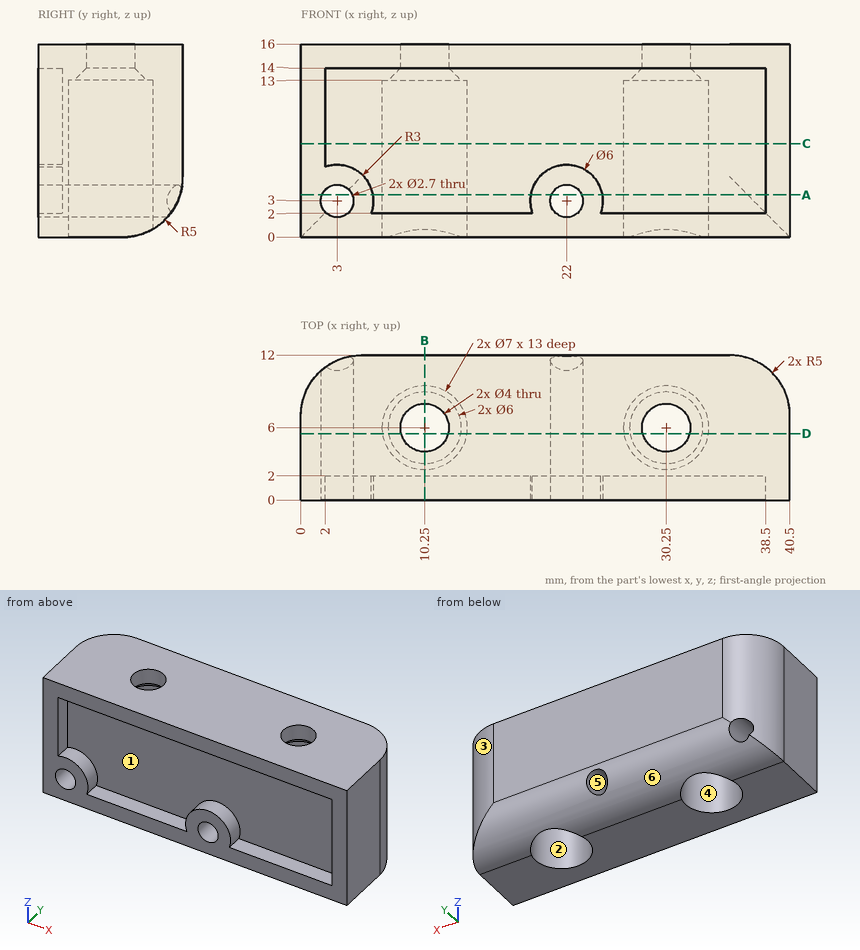
Job drawing, mm, ordinate dimensions from the low corner. One solid piece. A direction names the side the tool comes from. Round coordinates to 2 decimals unless told otherwise and drop trailing zeros. Write each loop counter-clockwise with the first axis right and the second up, starting at its lowest first coordinate (ties: lowest second). Pieces come first, ordered by that corner, then holes. Notation, with made-up numbers: M -21,-33.75 L 37,-33.75 A8 ccw 37,-27.75 Z; hole C 35.5,-12 d10. An arc over 180 degrees is marked long. Return JSON: item names as keys, results as strings. Group by question number.
(1) Two-plate mould, pull along Z, no slides. Class the marked faces 4, 5 and 6: +Z half, -Z half, draft (parallel to the pull), parting line (faces both ways), or undercut.
(2) Saw through at C-C on z = 7.75. Write the cut outline in (x, y), then the cut area to 3 significant figures.
(3) Drill centre lines: probe 1 along X at (y, z) = (1.25, 8); probe 2 along Y at (x, z) = (10.25, 8); probe 3 along X at (y, z) = (6.75, 4.5). Where is each one in solid material? Low to high.
(4) Saw through at D-D on y = 5.5. Count the separate pieces of the cut face and the enclosed holes in it, then the cut area to 3 significant figures.
(5) Saw through at A-A on z = 3.5. Write the cut outline in (x, y).
(6) Which spindle directions (+Z, -Z, +X, -X, +Y, -Y) get a long thin tool onto all of the face, cutting with end or side? Do the marked faces 1, 2 and 3. Say none if no direction does.
(7) Pin check, flat tips, straight feed: pin 1 Ø6.5 at (x, y) = (30.25, 6) entering from +Z; pin 2 Ø1 at (x, y) = (4, 9.5) entering from -Z; pin 3 Ø4.5 at (x, z) = (3, 3) entering from +Y; pin 4 Ø6 at (x, z) = (32, 7) entering from -Y. Stop position of each tip, or through.
(8) Saw through at B-B on x = 10.25. Write the cut outline in (y, z).
Returned:
{
 "1": {"face 4": "draft", "face 5": "undercut", "face 6": "-Z half"},
 "2": {"outline": "M 0,0 L 2,0 L 2,2 L 38.5,2 L 38.5,0 L 40.5,0 L 40.5,7 A5 ccw 35.5,12 L 5,12 A5 ccw 0,7 Z; hole C 10.25,6 d7; hole C 30.25,6 d7", "area": "325 mm²"},
 "3": {"probe 1": "0 to 2, 38.5 to 40.5", "probe 2": "2 to 2.5, 9.5 to 12", "probe 3": "0 to 6.83, 13.67 to 26.83, 33.67 to 40.5"},
 "4": {"separate pieces": "3", "enclosed holes": "2", "area": "431 mm²"},
 "5": {"outline": "M 0,0 L 1.75,0 L 1.75,10.8 A5 ccw 0,7 Z; M 4.25,0 L 5.96,0 L 5.96,2 L 19.04,2 L 19.04,0 L 20.75,0 L 20.75,11.77 L 4.25,11.77 Z; M 23.25,0 L 24.96,0 L 24.96,2 L 38.5,2 L 38.5,0 L 40.5,0 L 40.5,7 A5 ccw 37,11.77 L 23.25,11.77 Z; hole C 10.25,6 d7; hole C 30.25,6 d7"},
 "6": {"face 1": "-Y", "face 2": "-Z", "face 3": "+Z, -Z, +X, +Y"},
 "7": {"pin 1": "z = 16", "pin 2": "z = 0.42", "pin 3": "y = 11.98", "pin 4": "y = 2"},
 "8": {"outline": "M 0,0 L 2.5,0 L 2.5,13 L 3,13 L 4,14 L 4,16 L 0,16 L 0,14 L 2,14 L 2,2 L 0,2 Z; M 8,14 L 9,13 L 9.5,13 L 9.5,0.67 A5 ccw 12,5 L 12,16 L 8,16 Z"}
}
